For this review, take the finished solid that the model builds, in its own axes (mm). A direction names the side the tool comes from. Round coordinates to 2 decimals unless told otherwise and drop trailing zeros. Loops run counter-clockwise (first coordinate to the right, second up) from the corner with the lowest first, then second, coordinate; pieces in that order, holes last.
```python
from build123d import *

# Parameters (mm, degrees)
ESQUISSE1_W        = 45
ESQUISSE1_H        = 45
ESQUISSE1_R        = 16
BOSS_EXTRU_1_DEPTH = 5
ESQUISSE2_R        = 18.5
ESQUISSE2_R_2      = 16
BOSS_EXTRU_2_DEPTH = 20
ESQUISSE3_W        = 5
ESQUISSE3_H        = 4
BOSS_EXTRU_3_DEPTH = 3


with BuildPart() as part:
    # Esquisse1 → Boss.-Extru.1 (new body)
    with BuildSketch(Plane.XY):
        Rectangle(ESQUISSE1_W, ESQUISSE1_H)
        Circle(ESQUISSE1_R, mode=Mode.SUBTRACT)
    extrude(amount=BOSS_EXTRU_1_DEPTH)

    # Esquisse2 → Boss.-Extru.2 (add)
    with BuildSketch(Plane.XY.offset(5)):
        Circle(ESQUISSE2_R)
        Circle(ESQUISSE2_R_2, mode=Mode.SUBTRACT)
    extrude(amount=BOSS_EXTRU_2_DEPTH)

    # Esquisse3 → Boss.-Extru.3 (add)
    with BuildSketch(Plane(origin=(0, 0, 0), x_dir=(-1, 0, 0), z_dir=(0, 0, -1))):
        with Locations((16.5, 17)):
            Rectangle(ESQUISSE3_W, ESQUISSE3_H)
        with Locations((-16.5, 17)):
            Rectangle(ESQUISSE3_W, ESQUISSE3_H)
        with Locations((-16.5, -17)):
            Rectangle(ESQUISSE3_W, ESQUISSE3_H)
        with Locations((16.5, -17)):
            Rectangle(ESQUISSE3_W, ESQUISSE3_H)
    extrude(amount=BOSS_EXTRU_3_DEPTH)


solid = part.part
```
(1) Add section B-B (z = 2.5). Give the boundary of the cut face in (x, y).
(2) For L1, parallel to Y at x = 0, z = 11; L2, parallel to Z at x = -19, y = 20.5; L3, parallel to X at y = 13, z = 1, list the stretches that pass through material, from the lowest coordinate up.
(3) Add section D-D (y = -17). Give the boundary of the cut face in (x, z), plus the area to 3 significant figures.
(4) For faces 1 (the flat face through (-16, -19, -1)), 2 (the flat face through (20, 0, 5)), 3 (the flat face through (-16, 19, -1)), list the 3-axis set-ups (+Z, -Z, +X, -X, +Y, -Y) from which the entire face can be reached by the end or side of a thin tool; tool diameter is ignored.
(5) The part is to be moulded in two halves that separate along X. For faces 4 (the flat face through (19, -17, -1)), 5 (the flat face through (-14, 17, -1)), 6 (the cylindrical face through (-4.01, -18.06, 14.86)), 7 (the flat face through (14, 17, -1)), say which applies: pulls with the +X half, pulls with the -X half, needs draft (parallel to the pull), parting line crosses it, or undercut.
(6) Add section A-A (x = 0). Give the boundary of the cut face in (y, z).
(7) Insertion check: pin 1 Ø10 at (y, z) = (9.5, 15) entering from -X; pin 2 Ø2.5 at (y, z) = (-17, -2) entering from +X; pin 3 Ø2.5 at (x, z) = (17, -1.5) entering from -Y; pin 4 Ø13.5 at (x, y) = (-0.5, 2.5) entering from -Z. Each pin has a flat end and moves straight along its axis. Give the tip position at first contact, or say it passes through.
Outcome:
1. outline: (-22.5, -22.5) - (22.5, -22.5) - (22.5, 22.5) - (-22.5, 22.5) - close; hole circle Ø32 at (0, 0)
2. L1: y = -18.5 to -16, 16 to 18.5
2. L2: z = 0 to 5
2. L3: x = -22.5 to -9.33, 9.33 to 22.5
3. outline: (-22.5, 0) - (-19, 0) - (-19, -3) - (-14, -3) - (-14, 0) - (14, 0) - (14, -3) - (19, -3) - (19, 0) - (22.5, 0) - (22.5, 5) - (7.3, 5) - (7.3, 25) - (-7.3, 25) - (-7.3, 5) - (-22.5, 5) - close
3. area: 547 mm2
4. face 1: -Z, +X, -X, -Y
4. face 2: +Z
4. face 3: -Z, +X, -X, +Y
5. face 4: pulls with the +X half
5. face 5: undercut
5. face 6: parting line crosses it
5. face 7: undercut
6. outline: (-22.5, 0) - (-16, 0) - (-16, 25) - (-18.5, 25) - (-18.5, 5) - (-22.5, 5) - close; (16, 0) - (22.5, 0) - (22.5, 5) - (18.5, 5) - (18.5, 25) - (16, 25) - close
7. pin 1: stops at x = -17.94
7. pin 2: stops at x = 19
7. pin 3: stops at y = -19
7. pin 4: passes through
